Geometry: see drawing. Coordinates: mm, zero at the bounding-box minimum. Give positions to 0.01 mm unless a question says otherwise; leave off trailing zeros. Write item = value, one per line. Start each with the question number.
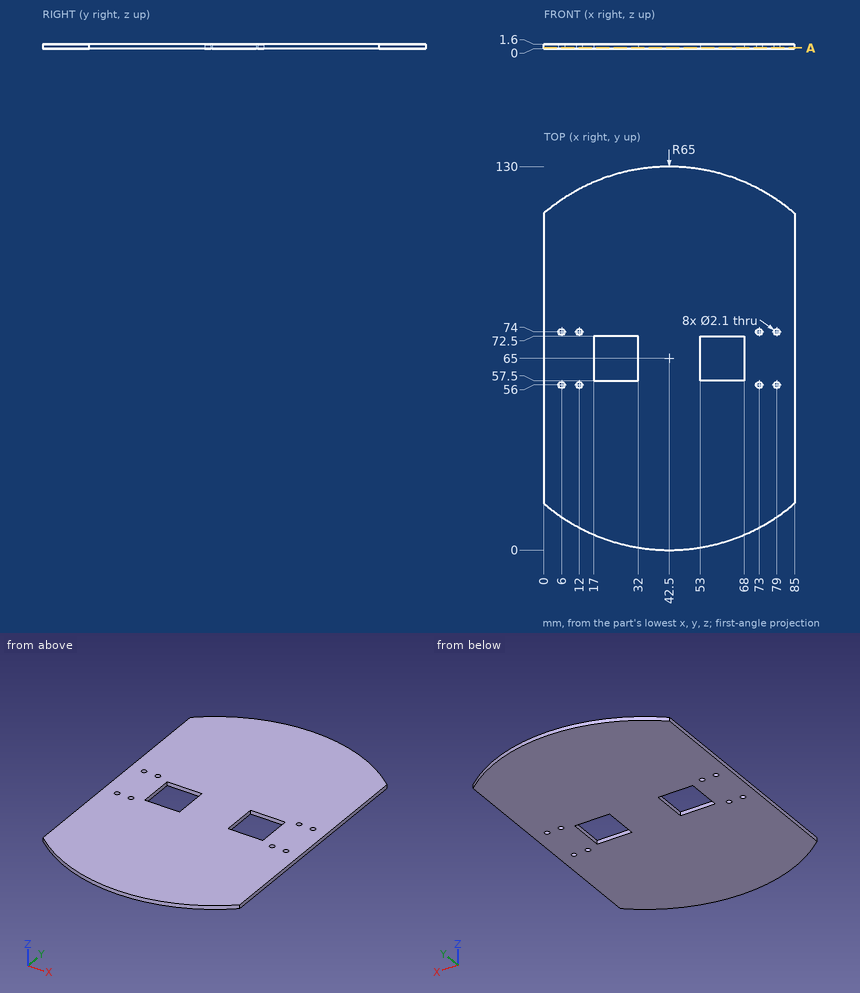
1) Pin query (flat end, axial travel): pin 1 Ø0.8 at (y, z) = (63.5, 0.5) entering from -X; pin 2 Ø0.8 at (x, z) = (64, 1) entering from +Y; pin 3 Ø0.5 at (x, z) = (21.5, 1) entering from -Y; pin 4 Ø0.8 at (x, z) = (58.5, 0.5) entering from -Y. Return the tip coordinate at first contact, or that it passes through.
2) Cut plane A-A (z = 0.25). Give the number of separate pieces and of enclosed holes in the cut face, plus the area to 3 significant figures.
3) Ray query, L1, parallel to Y at x = 79, z = 1.2; L2, parallel to Y at x = 12, z = 0.65; L3, parallel to Y at x = 29, z = 0.8. Return the intervals inside material, ascending.
Reply:
q1.pin_1 = 0
q1.pin_2 = 126.48
q1.pin_3 = 3.4
q1.pin_4 = 1.9
q2.separate_pieces = 1
q2.enclosed_holes = 10
q2.area = 9,720 mm²
q3.L1 = 11.22 to 54.95, 57.05 to 72.95, 75.05 to 118.78
q3.L2 = 7.6 to 54.95, 57.05 to 72.95, 75.05 to 122.4
q3.L3 = 1.42 to 57.5, 72.5 to 128.58
